Geometry: final body of the model. Coordinates: model frame, mm. Face numbers are marked on the shaded views. A direction names the side the tool comes from. Give positions to 0.01 mm unless a question says otherwise; leave off trailing zeros. Write each loop counter-clockwise with the first axis right and the second up, starting at its lowest first coordinate (ties: lowest second). Pieces come first, ordered by that corner, then holes.
from build123d import *

# Parameters (mm, degrees)
ESBO_O1_W                                      = 94
ESBO_O1_H                                      = 12
FLANGE_BASE1_DEPTH                             = 2
DOBRA_START                                    = -6
DOBRA_ESBO_ADA1_DEPTH                          = 12
DOBRA_ESBO_ADA1_2_DEPTH                        = 12
BROCA_DE_ROSQUEAR_DE_CANO_PARA_TARRAXA_D_D     = 3.3
BROCA_DE_ROSQUEAR_DE_CANO_PARA_TARRAXA_D_DEPTH = 4
BROCA_DE_ROSQUEAR_DE_CANO_PARA_TARRAXA_D_TIP   = 0.991420021


# Read off the part's stored shape, not the designer's step: Dobra esboçada1
# Sheet-metal steps are written as plain solids
with BuildPart() as part:
    # Esboço1 → Flange-base1 (new body)
    with BuildSketch(Plane.XY):
        Rectangle(ESBO_O1_W, ESBO_O1_H)
    extrude(amount=-FLANGE_BASE1_DEPTH)

    # Dobra esboçada1 outline → Dobra esboçada1 (cut)
    with BuildSketch(Plane(origin=(0, 0, 0), x_dir=(1, 0, 0), z_dir=(0, 1, 0)).offset(DOBRA_START)):
        with BuildLine():
            ThreePointArc((-36.464101616, 0), (-35, 1.464101615), (-33, 2))
            Line((-33, 2), (-47, 2))
            Line((-47, 2), (-47, 0))
            Line((-47, 0), (-36.464101616, 0))
        make_face()
        with BuildLine():
            Line((47, 2), (33, 2))
            ThreePointArc((33, 2), (35, 1.464101615), (36.464101616, 0))
            Line((36.464101616, 0), (47, 0))
            Line((47, 0), (47, 2))
        make_face()
    extrude(amount=DOBRA_ESBO_ADA1_DEPTH, mode=Mode.SUBTRACT)

    # Dobra esbo_ada1 2 outline → Dobra esbo_ada1 2 (add)
    with BuildSketch(Plane(origin=(0, 0, 0), x_dir=(1, 0, 0), z_dir=(0, 1, 0)).offset(DOBRA_START)):
        with BuildLine():
            Line((-33, 0), (-36.464101616, 0))
            ThreePointArc((-36.464101616, 0), (-36.863703305, -0.96472382), (-37, -2))
            Line((-37, -2), (-37, -11.28761102))
            Line((-37, -11.28761102), (-35, -11.28761102))
            Line((-35, -11.28761102), (-35, -2))
            ThreePointArc((-35, -2), (-34.414213562, -0.585786438), (-33, 0))
        make_face()
        with BuildLine():
            ThreePointArc((37, -2), (36.863703305, -0.96472382), (36.464101616, 0))
            Line((36.464101616, 0), (33, 0))
            ThreePointArc((33, 0), (34.414213562, -0.585786438), (35, -2))
            Line((35, -2), (35, -11.28761102))
            Line((35, -11.28761102), (37, -11.28761102))
            Line((37, -11.28761102), (37, -2))
        make_face()
    extrude(amount=DOBRA_ESBO_ADA1_2_DEPTH)

    # Broca de rosquear de cano para tarraxa de 1/81
    with Locations(Plane(origin=(0, 0, -2), x_dir=(-1, 0, 0), z_dir=(0, 0, -1))):
        with Locations((0, 0)):
            Hole(BROCA_DE_ROSQUEAR_DE_CANO_PARA_TARRAXA_D_D / 2, depth=BROCA_DE_ROSQUEAR_DE_CANO_PARA_TARRAXA_D_DEPTH)
            with Locations((0, 0, -(BROCA_DE_ROSQUEAR_DE_CANO_PARA_TARRAXA_D_DEPTH + BROCA_DE_ROSQUEAR_DE_CANO_PARA_TARRAXA_D_TIP / 2))):  # 118° drill point
                Cone(0, BROCA_DE_ROSQUEAR_DE_CANO_PARA_TARRAXA_D_D / 2, BROCA_DE_ROSQUEAR_DE_CANO_PARA_TARRAXA_D_TIP, mode=Mode.SUBTRACT)


solid = part.part
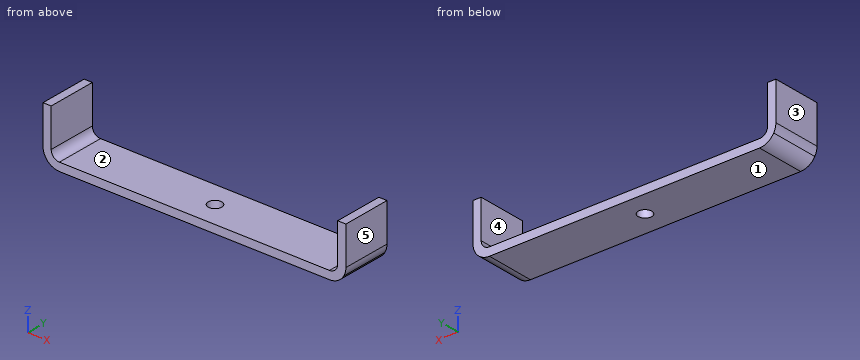
Q1. Section B-B on x = 0. Output: boundary loops of the cut face in (y, z), plus the area to 3 significant figures.
Filled sheet:
outline: (-6, -2) - (-1.65, -2) - (-1.65, 0) - (-6, 0) - close; (1.65, -2) - (6, -2) - (6, 0) - (1.65, 0) - close
area: 17.4 mm2
Q2. Pull-direction query (X, two-part tool) for the marked faces 3, 4 and 5; classes: released by +X, released by -X, zero draft, split by the parting line, or undercut.
Filled sheet:
face 3: released by -X
face 4: undercut
face 5: released by +X
Q3. Section A-A on z = 4. Output: boundary loops of the cut face in (x, y), plus the area to 3 significant figures.
Filled sheet:
outline: (-37, -6) - (-35, -6) - (-35, 6) - (-37, 6) - close; (35, -6) - (37, -6) - (37, 6) - (35, 6) - close
area: 48.0 mm2
Q4. Access query for the marked faces 1 and 2. Directions: +Z, -Z, +X, -X, +Y, -Y. A direction counts if a zero-diameter tool reaches every point of the face in a straight line with its end or side. Return the directions, or none.
Filled sheet:
face 1: -Z, +X, -X, +Y, -Y
face 2: +Z, +Y, -Y
Q5. Ray query, line 1 along Y through (x, z) = (0, -1.15); line 2 along X through (y, z) = (-5, 10.25); line 3 along Z through (x, y) = (-14, -5). Return the intervals inside material, ascending.
Filled sheet:
line 1: y = -6 to -1.65, 1.65 to 6
line 2: x = -37 to -35, 35 to 37
line 3: z = -2 to 0
Q6. Section D-D on y = -5. Output: boundary loops of the cut face in (x, z), plus the area to 3 significant figures.
Filled sheet:
outline: (-37, 2) arc R4 ccw to (-33, -2) - (33, -2) arc R4 ccw to (37, 2) - (37, 11.29) - (35, 11.29) - (35, 2) arc R2 cw to (33, 0) - (-33, 0) arc R2 cw to (-35, 2) - (-35, 11.29) - (-37, 11.29) - close
area: 188 mm2
Q7. Pin query (flat end, axial travel): P1, Ø6, axis at x = 2, y = -3, coming from the +Z side. Return the tip coordinate at first contact, or that it passes through.
Filled sheet:
P1: stops at z = 0
Q8. Section C-C on y = 0. Output: boundary loops of the cut face in (x, z).
Filled sheet:
outline: (-37, 2) arc R4 ccw to (-33, -2) - (-1.65, -2) - (-1.65, 0) - (-33, 0) arc R2 cw to (-35, 2) - (-35, 11.29) - (-37, 11.29) - close; (1.65, -2) - (33, -2) arc R4 ccw to (37, 2) - (37, 11.29) - (35, 11.29) - (35, 2) arc R2 cw to (33, 0) - (1.65, 0) - close
